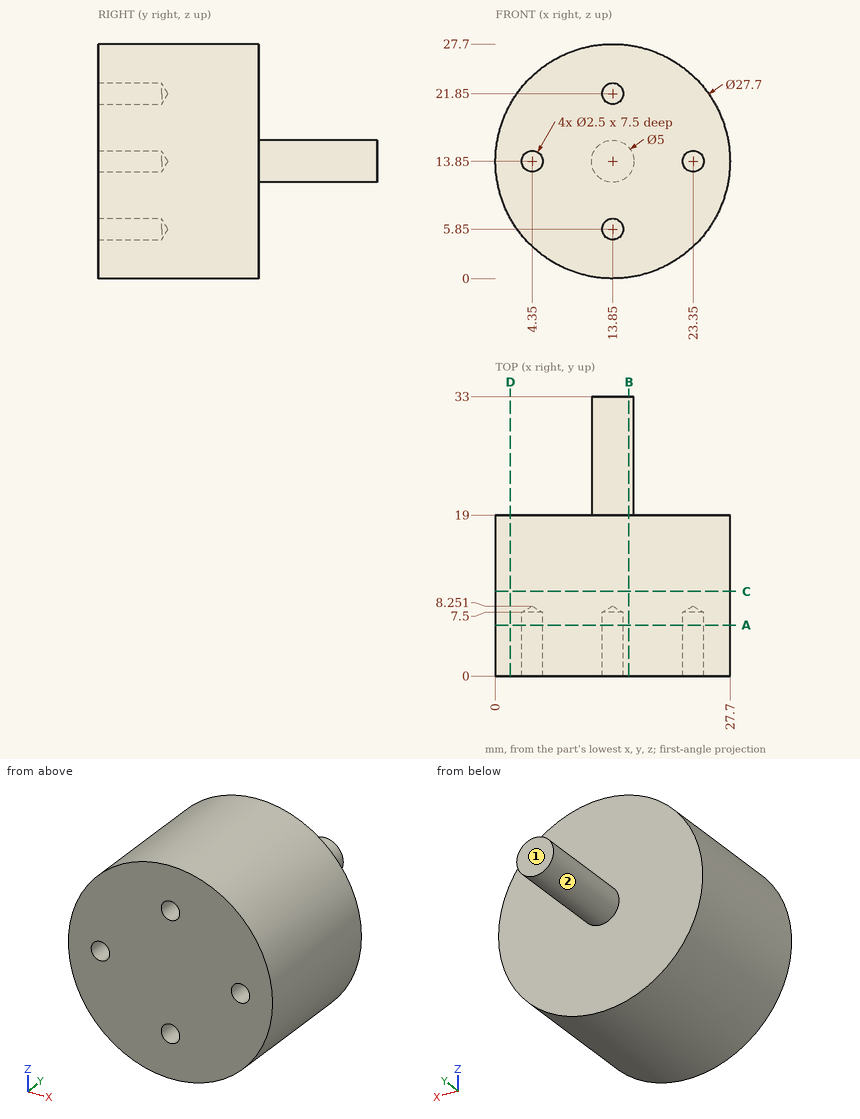
Design review of the part shown in the three views and the two pictorial views. Dimensions are in mm from the part's minimum x, y and z. A direction names the side the tool comes from. Round coordinates to 2 decimals unless told otherwise and drop trailing zeros. Write each loop counter-clockwise with the first axis right and the second up, starting at its lowest first coordinate (ties: lowest second). Pieces come first, ordered by that corner, then holes.
Item 1: We need section C-C on y = 10. Write out the cut boundary in (x, z), and give its area (3 significant figures).
Item 2: For the marked faces 1 and 2, list the 3-axis set-ups (+Z, -Z, +X, -X, +Y, -Y) from which the entire face can be reached by the end or side of a thin tool; tool diameter is ignored.
Item 3: For probe 1 along X at (y, z) = (3.75, 13.85); probe 2 along Z at (x, y) = (13.85, 4); probe 3 along Y at (x, z) = (23, 8), list the stretches that pass through material, from the lowest coordinate up.
Item 4: We need section D-D on x = 1.75. Write out the cut boundary in (y, z).
Item 5: We need section A-A on y = 6. Write out the cut boundary in (x, z), and give its area (3 significant figures).
Item 6: We need section B-B on x = 15.75. Write out the cut boundary in (y, z), and give its area (3 significant figures).
Item 7: Clearance check with flat-ended pins moving along their axes: pin 1 Ø1 at (x, y) = (24, 8) entering from -Z (1 decimal); pin 2 Ø4 at (y, z) = (7, 9.5) entering from -X; pin 3 Ø1.5 at (x, z) = (13.85, 5.85) entering from -Y. State where each tip first meets the part, or that it passes through.
Returned:
1. outline: circle Ø27.7 at (13.85, 13.85)
1. area: 603 mm2
2. face 1: +Z, -Z, +X, -X, +Y
2. face 2: +Y
3. probe 1: x = 0 to 3.1, 5.6 to 22.1, 24.6 to 27.7
3. probe 2: z = 0 to 4.6, 7.1 to 20.6, 23.1 to 27.7
3. probe 3: y = 0 to 19
4. outline: (0, 7.11) - (19, 7.11) - (19, 20.59) - (0, 20.59) - close
5. outline: circle Ø27.7 at (13.85, 13.85); hole circle Ø2.5 at (4.35, 13.85); hole circle Ø2.5 at (13.85, 5.85); hole circle Ø2.5 at (13.85, 21.85); hole circle Ø2.5 at (23.35, 13.85)
5. area: 583 mm2
6. outline: (0, 0.13) - (19, 0.13) - (19, 12.23) - (33, 12.23) - (33, 15.47) - (19, 15.47) - (19, 27.57) - (0, 27.57) - close
6. area: 567 mm2
7. pin 1: stops at z = 3.9
7. pin 2: stops at x = 0.2
7. pin 3: stops at y = 7.8
